Read the model definition and answer for the solid it produces. Units are mm, in the model's axes. Coordinates: 2 decimals unless noted, no trailing zeros. Order: outer loops, then holes, each group sorted by start corner. A loop starts at its lowest first (then second) coordinate and runs counter-clockwise, first axis right, second up. Notation, with made-up numbers: M 4,28.5 L 40,28.5 A20 ccw 40,43.5 Z; hole C 54.25,52.25 d7. An arc over 180 degrees is marked long. Write each question's results on one line, items separated by ' | '.
```python
from build123d import *

# Parameters (mm, degrees)
SKETCH_1_R      = 4
EXTRUDE_1_DEPTH = 5


with BuildPart() as part:
    # 草图1 → 凸台-拉伸1 (new body)
    with BuildSketch(Plane.XY):
        Polygon((10, -10), (40, -10), (60, -10), (60, 10), (40, 10), (10, 10), (-10, 10), (-10, -10), align=None)
        Circle(SKETCH_1_R, mode=Mode.SUBTRACT)
        with Locations((50, 0)):
            Circle(SKETCH_1_R, mode=Mode.SUBTRACT)
    extrude(amount=EXTRUDE_1_DEPTH)


solid = part.part
```
(1) Given pin 1 (9 mm diameter, centred on x = 0, y = 0, fed in from -Z), flat-ended and moving along its own axis, determine where the tip first touches the part or whether it passes through.
Conclusion:
pin 1: z = 0
(2) The mould has two halves that part along X. Classify faces 1 (the flat face through (-10, 0, 2)), 2 (the flat face through (60, 0, 2)), 3 (the flat face through (25, -10, 2)), 4 (the cylindrical face through (46, 0, 2)): pulls with the +X half, pulls with the -X half, needs draft (parallel to the pull), parting line crosses it, or undercut.
Conclusion:
face 1: pulls with the -X half | face 2: pulls with the +X half | face 3: needs draft | face 4: undercut
(3) The part is cut by section C-C, the plane z = 1. Write down the section's boundary in (x, y), then the cut area to 3 significant figures.
Conclusion:
outline: M -10,-10 L 60,-10 L 60,10 L -10,10 Z; hole C 0,0 d8; hole C 50,0 d8 | area: 1,300 mm²
(4) The part is cut by section A-A, the plane x = 0. Write down the section's boundary in (y, z), then the cut area to 3 significant figures.
Conclusion:
outline: M -10,0 L -4,0 L -4,5 L -10,5 Z; M 4,0 L 10,0 L 10,5 L 4,5 Z | area: 60.0 mm²
(5) The part is cut by section B-B, the plane y = 0. Write down the section's boundary in (x, z).
Conclusion:
outline: M -10,0 L -4,0 L -4,5 L -10,5 Z; M 4,0 L 46,0 L 46,5 L 4,5 Z; M 54,0 L 60,0 L 60,5 L 54,5 Z
(6) Straight lines are drawn through the part: line 1 (X direction, y = -0.25, z = 2.85); line 2 (Y direction, x = 50, z = 1.15); line 3 (Y direction, x = 48.5, z = 0.25). For each, find the intervals that lie inside material, in ascending order.
Conclusion:
line 1: -10 to -3.99, 3.99 to 46.01, 53.99 to 60 | line 2: -10 to -4, 4 to 10 | line 3: -10 to -3.71, 3.71 to 10
